For this review, use the dimensioned drawing (mm, ordinates from the lowest corner) and the shaded views. A direction names the side the tool comes from. Round coordinates to 2 decimals unless told otherwise and drop trailing zeros. Order: outer loops, then holes, each group sorted by start corner. A loop starts at its lowest first (then second) coordinate and runs counter-clockwise, first axis right, second up. Notation, with made-up numbers: M 6,10 L 32,10 A17 cw 32,39 Z; hole C 60,-5.75 d7. An arc over 180 degrees is marked long. Use a Markdown table: item, result. Add a question column.
1. Consider section A-A on y = 5. State the section outline as (x, z) points, then the cut area to 3 significant figures.
2. Consider section D-D on z = 21. State the section outline as (x, y) points, then the cut area to 3 significant figures.
3. For the marked faces 1 and 2, list the 3-axis set-ups (+Z, -Z, +X, -X, +Y, -Y) from which the entire face can be reached by the end or side of a thin tool; tool diameter is ignored.
4. Consider section C-C on z = 24.9. State the section outline as (x, y) points, then the cut area to 3 significant figures.
5. To check wall thickness, follow probe 1 along Y at (x, z) = (5.5, 11.5); probe 2 along X at (y, z) = (9.55, 24.9); probe 3 along Z at (x, y) = (15, 5.5). State the ranges of each line that lie inside material, in increasing order.
6. Insertion check: P1, Ø4.5, axis at x = 15, z = 24.9, coming from the +Y side. The pin has a flat end and moves straight along its axis. Give the tip position at first contact, or say it passes through.
7. Consider section B-B on x = 5.5. State the section outline as (y, z) points.
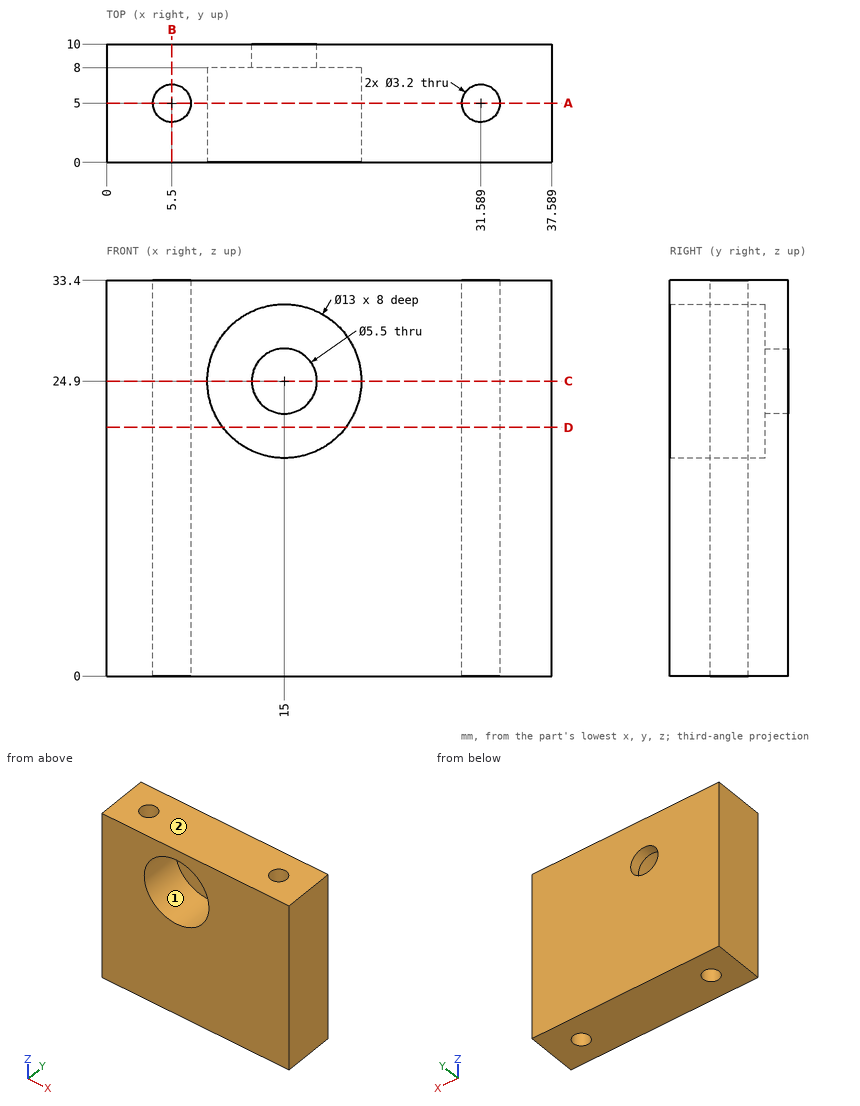
Answer block:
| question | item | result |
|---|---|---|
| 1 | outline | M 0,0 L 3.9,0 L 3.9,33.4 L 0,33.4 Z; M 7.1,0 L 29.99,0 L 29.99,33.4 L 7.1,33.4 Z; M 33.19,0 L 37.59,0 L 37.59,33.4 L 33.19,33.4 Z; hole C 15,24.9 d13 |
| 1 | area | 909 mm^2 |
| 2 | outline | M 0,0 L 9.8,0 L 9.8,8 L 20.2,8 L 20.2,0 L 37.59,0 L 37.59,10 L 0,10 Z; hole C 5.5,5 d3.2; hole C 31.59,5 d3.2 |
| 2 | area | 277 mm^2 |
| 3 | face 1 | -Y |
| 3 | face 2 | +Z, +X, -X, +Y, -Y |
| 4 | outline | M 0,0 L 8.5,0 L 8.5,8 L 12.25,8 L 12.25,10 L 0,10 Z; M 17.75,8 L 21.5,8 L 21.5,0 L 37.59,0 L 37.59,10 L 17.75,10 Z; hole C 5.5,5 d3.2; hole C 31.59,5 d3.2 |
| 4 | area | 245 mm^2 |
| 5 | probe 1 | 0 to 3.4, 6.6 to 10 |
| 5 | probe 2 | 0 to 12.25, 17.75 to 37.59 |
| 5 | probe 3 | 0 to 18.4, 31.4 to 33.4 |
| 6 | P1 | through |
| 7 | outline | M 0,0 L 3.4,0 L 3.4,33.4 L 0,33.4 Z; M 6.6,0 L 10,0 L 10,33.4 L 6.6,33.4 Z |
